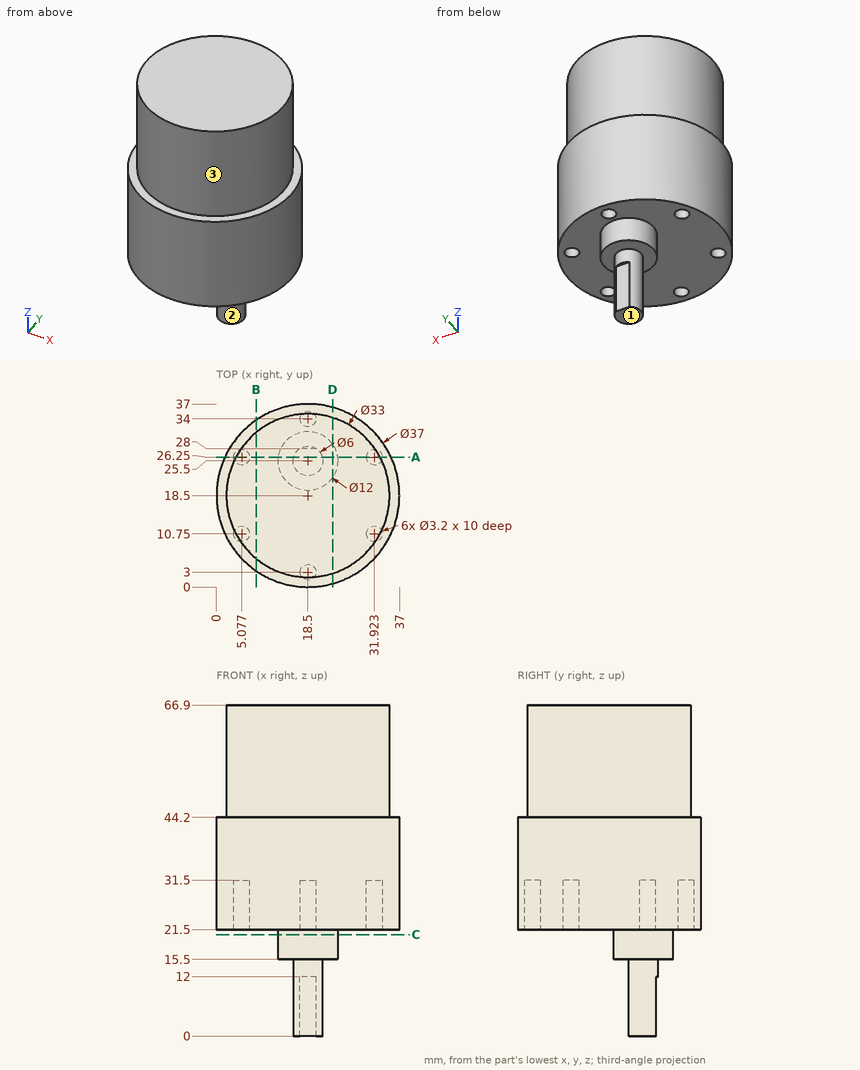
For this review, use the dimensioned drawing (mm, ordinates from the lowest corner) and the shaded views. A direction names the side the tool comes from. Round coordinates to 2 decimals unless told otherwise and drop trailing zeros. Order: outer loops, then holes, each group sorted by start corner. A loop starts at its lowest first (then second) coordinate and runs counter-clockwise, first axis right, second up.
1) Consider section C-C (z = 20.5). State the section outline as (x, y) points.
The answers:
outline: circle Ø12 at (18.5, 25.5)
2) Clearance check with flat-ended pins moving along their axes: pin 1 Ø3 at (y, z) = (22.5, 59) entering from -X; pin 2 Ø1 at (y, z) = (26, 35) entering from -X (1 decimal); pin 3 Ø3.5 at (x, y) = (32.5, 26.5) entering from -Z. State where each tip first meets the part, or that it passes through.
The answers:
pin 1: stops at x = 2.19
pin 2: stops at x = 1.4
pin 3: stops at z = 21.5
3) Consider section B-B (x = 8). State the section outline as (y, z) points.
The answers:
outline: (3.27, 21.5) - (33.73, 21.5) - (33.73, 44.2) - (31.23, 44.2) - (31.23, 66.9) - (5.77, 66.9) - (5.77, 44.2) - (3.27, 44.2) - close
4) For L1, parallel to Y at x = 18.5, z = 26.75; L2, parallel to Y at x = 6, z = 23 (1 decimal); L3, parallel to X at y = 7, z = 50, list the stretches that pass through material, from the lowest coordinate up.
The answers:
L1: y = 0 to 1.4, 4.6 to 32.4, 35.6 to 37
L2: y = 4.9 to 9.4, 12.1 to 24.9, 27.6 to 32.1
L3: x = 6.67 to 30.33
5) Consider section A-A (y = 26.25). State the section outline as (x, z) points (1 decimal), plus the area to 3 significant figures.
The answers:
outline: (1.7, 21.5) - (3.5, 21.5) - (3.5, 31.5) - (6.7, 31.5) - (6.7, 21.5) - (12.5, 21.5) - (12.5, 15.5) - (15.6, 15.5) - (15.6, 0) - (21.4, 0) - (21.4, 15.5) - (24.5, 15.5) - (24.5, 21.5) - (30.3, 21.5) - (30.3, 31.5) - (33.5, 31.5) - (33.5, 21.5) - (35.3, 21.5) - (35.3, 44.2) - (33.1, 44.2) - (33.1, 66.9) - (3.9, 66.9) - (3.9, 44.2) - (1.7, 44.2) - close
area: 1,520 mm2
6) Machinability: for the marked faces 1, 2 and 3, which of the approach directions +Z, -Z, +X, -X, +Y, -Y give a long, thin tool a straight path to every point of the face, cutting with its end or side? Answer none if there is none.
The answers:
face 1: -Z, +X, -X, +Y, -Y
face 2: -Z
face 3: +Z
7) Consider section D-D (x = 23.5). State the section outline as (y, z) points, plus the area to 3 significant figures.
The answers:
outline: (0.69, 21.5) - (22.18, 21.5) - (22.18, 15.5) - (28.82, 15.5) - (28.82, 21.5) - (36.31, 21.5) - (36.31, 44.2) - (34.22, 44.2) - (34.22, 66.9) - (2.78, 66.9) - (2.78, 44.2) - (0.69, 44.2) - close
area: 1,560 mm2
